from build123d import *

# Parameters (mm, degrees)
F0_W     = 304.8
F0_H     = 228.6
F1_DEPTH = 304.8
F2_W     = 208.28
F2_H     = 284.48
F3_DEPTH = 294.64
F4_R     = 38.1
F5_DEPTH = 25.4


with BuildPart() as f1:
    # F0 (on Top) → F1 (new body)
    with BuildSketch(Plane.XY):
        Rectangle(F0_W, F0_H)
    extrude(amount=F1_DEPTH)

    # F2 (on face) → F3 (cut)
    with BuildSketch(Plane(origin=(-152.4, 0, 0), x_dir=(0, -1, 0), z_dir=(-1, 0, 0))):
        with Locations((0, 152.4)):
            Rectangle(F2_W, F2_H)
    extrude(amount=-F3_DEPTH, mode=Mode.SUBTRACT)

    # F4 (on face) → F5 (cut)
    with BuildSketch(Plane.YZ.offset(152.4)):
        with Locations((0, 152.4)):
            Circle(F4_R)
    extrude(amount=-F5_DEPTH, mode=Mode.SUBTRACT)


solid = f1.part
Can you work these out from the model? Positions are in its coordinate system, mm. A direction names the side the tool comes from. Give positions to 0.01 mm unless a question says otherwise; leave off trailing zeros. Order: outer loops, then holes, each group sorted by start corner. A loop starts at its lowest first (then second) coordinate and runs counter-clockwise, first axis right, second up. Notation, with made-up numbers: M -6.75,64 L 23.25,64 A5 ccw 23.25,72 Z; hole C -8.5,13.5 d6. An arc over 180 degrees is marked long. Use a Markdown table: item, result. Add a question column.
Item 1: If I drill on L1, parallel to Y at x = 74.5, z = 64.5; L2, parallel to Z at x = 150, y = 0; L3, parallel to Z at x = 57.5, y = 9.5, over which ranges is the centre line in solid material (lowest first)? Write a range as [from, to].
Item 2: We'd pull the mould along Y, two halves only. Please class faces 1 (the cylindrical face through (147.391, -4.96, 190.176)), 2 (the flat face through (-2, -114.3, 150)), 3 (the flat face through (-152.4, -111, 152)): +Y half, -Y half, draft (parallel to the pull), parting line (faces both ways), or undercut.
Item 3: Suppose I cut it at A-A (z = 152.4). List the corners of the cut face in (x, y) for me.
Item 4: Will this pin go through, and if not, where does the flat tip stop? pin 1 (10 mm diameter, centred on y = -42, z = 170, fed in from -X).
Item 5: Suppose I cut it at B-B (y = 0). List the corners of the cut face in (x, z) for me, then the cut area to 3 significant figures.
Item 6: For faces 4 (the flat face through (152.4, 24, 184)), 5 (the flat face through (-7, 1, 10.16)), which set-ups out of +Z, -Z, +X, -X, +Y, -Y let a thin tool reach every point of the face, with its end or its side?
Item 7: Suppose I cut it at C-C (x = 22). List the corners of the cut face in (y, z) for me, then the cut area to 3 significant figures.
Item 8: Suppose I cut it at D-D (z = 272). List the corners of the cut face in (x, y) for me.
Answer sheet:
| question | item | result |
|---|---|---|
| 1 | L1 | y = [-114.3, -104.14], [104.14, 114.3] |
| 1 | L2 | z = [0, 114.3], [190.5, 304.8] |
| 1 | L3 | z = [0, 10.16], [294.64, 304.8] |
| 2 | face 1 | undercut |
| 2 | face 2 | -Y half |
| 2 | face 3 | draft |
| 3 | outline | M -152.4,-114.3 L 152.4,-114.3 L 152.4,-38.1 L 142.24,-38.1 L 142.24,-104.14 L -152.4,-104.14 Z; M -152.4,104.14 L 142.24,104.14 L 142.24,38.1 L 152.4,38.1 L 152.4,114.3 L -152.4,114.3 Z |
| 4 | pin 1 | stops at x = 142.24 |
| 5 | outline | M -152.4,0 L 152.4,0 L 152.4,114.3 L 142.24,114.3 L 142.24,10.16 L -152.4,10.16 Z; M -152.4,294.64 L 142.24,294.64 L 142.24,190.5 L 152.4,190.5 L 152.4,304.8 L -152.4,304.8 Z |
| 5 | area | 8,310 mm² |
| 6 | face 4 | +Z, -Z, +X, +Y, -Y |
| 6 | face 5 | -X |
| 7 | outline | M -114.3,0 L 114.3,0 L 114.3,304.8 L -114.3,304.8 Z; hole M -104.14,10.16 L 104.14,10.16 L 104.14,294.64 L -104.14,294.64 Z |
| 7 | area | 10,400 mm² |
| 8 | outline | M -152.4,-114.3 L 152.4,-114.3 L 152.4,114.3 L -152.4,114.3 L -152.4,104.14 L 142.24,104.14 L 142.24,-104.14 L -152.4,-104.14 Z |
